```python
from build123d import *

# Parameters (mm, degrees)
SKETCH1_W           = 15
SKETCH1_H           = 15
BOSS_EXTRUDE1_DEPTH = 5
BOSS_EXTRUDE2_DEPTH = 5
SKETCH3_R           = 4
BOSS_EXTRUDE3_DEPTH = 10


with BuildPart() as part:
    # Sketch1 → Boss-Extrude1 (new body)
    with BuildSketch(Plane(origin=(0, 0, 0), x_dir=(1, 0, 0), z_dir=(0, 1, 0))):
        Rectangle(SKETCH1_W, SKETCH1_H)
    extrude(amount=BOSS_EXTRUDE1_DEPTH)

    # Sketch2 → Boss-Extrude2 (add)
    with BuildSketch(Plane(origin=(0, 5, 0), x_dir=(1, 0, 0), z_dir=(0, 1, 0))):
        Polygon((-2.886751346, 5), (-5.773502692, 0), (-2.886751346, -5), (2.886751346, -5), (5.773502692, 0), (2.886751346, 5), align=None)
    extrude(amount=BOSS_EXTRUDE2_DEPTH)

    # Sketch3 → Boss-Extrude3 (add)
    with BuildSketch(Plane.XZ):
        with Locations(Location((0, 0, 0), (0, 0, 270))):
            Circle(SKETCH3_R)
    extrude(amount=BOSS_EXTRUDE3_DEPTH)


solid = part.part
```
Input: part model. Units: mm. Frame: model coordinates. A direction names the side the tool comes from. Coordinates: 2 decimals unless noted, no trailing zeros. Write each loop counter-clockwise with the first axis right and the second up, starting at its lowest first coordinate (ties: lowest second). Pieces come first, ordered by that corner, then holes. Notation, with made-up numbers: (-33, 72) - (22, 72) arc R25 cw to (22, 99) - close; hole circle Ø4 at (59, 59.5). An arc over 180 degrees is marked (long way). Put each result on its own line as item: value. Start each with the question number.
1) Reachability of faces 1 (the face through (-4.35, 7.465, 2.465)), 2 (the face through (0, 7, -5)), 3 (the face through (-3.905, -4.93, 0.867)), 4 (the face through (4.31, 7.465, 2.535)) from +Z, -Z, +X, -X, +Y, -Y: full face, straight path, thin tool, end or side. Return the list, or none.
2) Cut plane D-D (y = -2.75). Return the cut outline in (x, z), plus the area to 3 significant figures.
3) Cut plane C-C (z = 1.5). Return the cut outline in (x, y).
4) Contact query for flat-ended pins moving along their axis: pin 1 (2.5 mm diameter, centred on x = 1.5, y = 7, fed in from +Z); pin 2 (6 mm diameter, centred on x = 5.5, y = -8, fed in from -Z). Output: stop coordinate, or through.
5) Cut plane B-B (y = 8.25). Return the cut outline in (x, z), plus the area to 3 significant figures.
6) Ray query, L1, parallel to Y at x = 0, z = -5.75; L2, parallel to Z at x = 0, y = 6; L3, parallel to Y at x = -3.25, z = -3.75. Return the intervals inside material, ascending.
7) Cut plane A-A (x = 0). Return the cut outline in (y, z), plus the area to 3 significant figures.
Resolved:
1. face 1: +Z, -X, +Y
1. face 2: -Z, +X, -X, +Y
1. face 3: -Y
1. face 4: +Z, +X, +Y
2. outline: circle Ø8 at (0, 0)
2. area: 50.3 mm2
3. outline: (-7.5, 0) - (-3.71, 0) - (-3.71, -10) - (3.71, -10) - (3.71, 0) - (7.5, 0) - (7.5, 5) - (4.91, 5) - (4.91, 10) - (-4.91, 10) - (-4.91, 5) - (-7.5, 5) - close
4. pin 1: stops at z = 5
4. pin 2: stops at z = -3.12
5. outline: (-5.77, 0) - (-2.89, -5) - (2.89, -5) - (5.77, 0) - (2.89, 5) - (-2.89, 5) - close
5. area: 86.6 mm2
6. L1: y = 0 to 5
6. L2: z = -5 to 5
6. L3: y = 0 to 10
7. outline: (-10, -4) - (0, -4) - (0, -7.5) - (5, -7.5) - (5, -5) - (10, -5) - (10, 5) - (5, 5) - (5, 7.5) - (0, 7.5) - (0, 4) - (-10, 4) - close
7. area: 205 mm2
